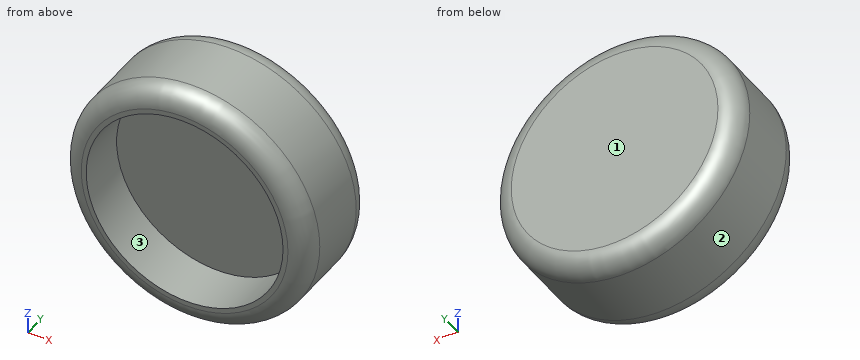
Autodesk Inventor part; units mm, degrees
ref_plane "YZ Plane" through (0, 0, 0) normal (1, 0, 0) x (0, 1, 0)
ref_plane "XZ Plane" through (0, 0, 0) normal (0, 1, 0) x (-1, 0, 0)
ref_plane "XY Plane" through (0, 0, 0) normal (0, 0, 1) x (1, 0, 0)
sketch "Sketch1" plane through (0, 0, 0) normal (0, 1, 0) x (-1, 0, 0)
  circle A0 centre (0, 0) radius 12.5
  dimension "d0" = 25
extrude "Extrusion1" add sketch "Sketch1" along normal blind 10
sketch "Sketch2" plane through (0, 0, 0) normal (0, -1, 0) x (1, 0, 0)
  circle A0 centre (0, 0) radius 10
  dimension "d3" = 20
extrude "Extrusion2" cut sketch "Sketch2" against normal blind 5
fillet "Fillet1" radius 2 2 edges at (12.5, 10, 0) (12.5, 0, 0)
sketch "Sketch3" plane through (0, 0, 0) normal (0, 0, 1) x (1, 0, 0)
  point P0 (0, 0)
sketch "Sketch4" plane through (0, 5, 0) normal (0, -1, 0) x (1, 0, 0)
  point P0 (0, 0)
equation "\"BendRadius\" = Thickness"
equation "\"BendReliefWidth\" = Thickness"
equation "\"BendReliefDepth\" = 0.5 * Thickness"
equation "\"CornerReliefSize\" = 4 * Thickness"
equation "\"MinimumRemnant\" = 2 * Thickness"
equation "\"TransitionRadius\" = BendRadius"
equation "\"JacobiRadiusSize\" = BendRadius"
equation "\"GapSize\" = Thickness"
Can you work these out from the model? Positions are in its coordinate system, mm. Face numbers are marked on the shaded views. Coordinates: 2 decimals unless noted, no trailing zeros. Loops run counter-clockwise (first coordinate to the right, second up) from the corner with the lowest first, then second, coordinate; pieces in that order, holes last. Notation, with made-up numbers: M 70,58 L 117,58 A13 ccw 117,76 Z; hole C 38.5,26 d10. An arc over 180 degrees is marked long. Answer as CSV lines item,"result". Start each with the question number.
1. Thinking about a two-plate mould opening in X: for the marked faces 1, 2 and 3, which applies, +X half, -X half, draft (parallel to the pull), parting line (faces both ways), or undercut?
2. Suppose I cut it at C-C, the plane y = 6.5. List the corners of the cut face in (x, z) for me, plus the area to 3 significant figures.
3. If I drill on probe 1 along Z at (x, y) = (0, 3.3); probe 2 along Y at (x, z) = (-8, -0.5); probe 3 along Z at (x, y) = (2.75, 2), over which ranges is the centre line in solid material (lowest first)? Write a range as [from, to].
4. For pin 1 Ø10 at (x, z) = (2.5, 0) entering from -Y; pin 2 Ø12 at (x, z) = (1, 9) entering from -Y; pin 3 Ø5 at (x, y) = (-3.5, 4) entering from -Z; pin 4 Ø5 at (y, z) = (2, 8.5) entering from -X, each with a flat end and sliding along its axis, tell me the tip position at first contact or that it passes through.
5. Suppose I cut it at B-B, the plane z = 0. List the corners of the cut face in (x, y) for me.
6. Suppose I cut it at A-A, the plane x = 0. List the corners of the cut face in (y, z) for me.
Output:
1,face 1,"draft"
1,face 2,"parting line"
1,face 3,"undercut"
2,outline,"C 0,0 d25"
2,area,"491 mm^2"
3,probe 1,"z = [-12.5, -10], [10, 12.5]"
3,probe 2,"y = [5, 10]"
3,probe 3,"z = [-12.19, -9.61], [9.61, 12.19]"
4,pin 1,"stops at y = 5"
4,pin 2,"stops at y = 0"
4,pin 3,"stops at z = -12.46"
4,pin 4,"stops at x = -10.97"
5,outline,"M -12.5,2 A2 ccw -10.5,0 L -10,0 L -10,5 L 10,5 L 10,0 L 10.5,0 A2 ccw 12.5,2 L 12.5,8 A2 ccw 10.5,10 L -10.5,10 A2 ccw -12.5,8 Z"
6,outline,"M 0,-10.5 A2 ccw 2,-12.5 L 8,-12.5 A2 ccw 10,-10.5 L 10,10.5 A2 ccw 8,12.5 L 2,12.5 A2 ccw 0,10.5 L 0,10 L 5,10 L 5,-10 L 0,-10 Z"
